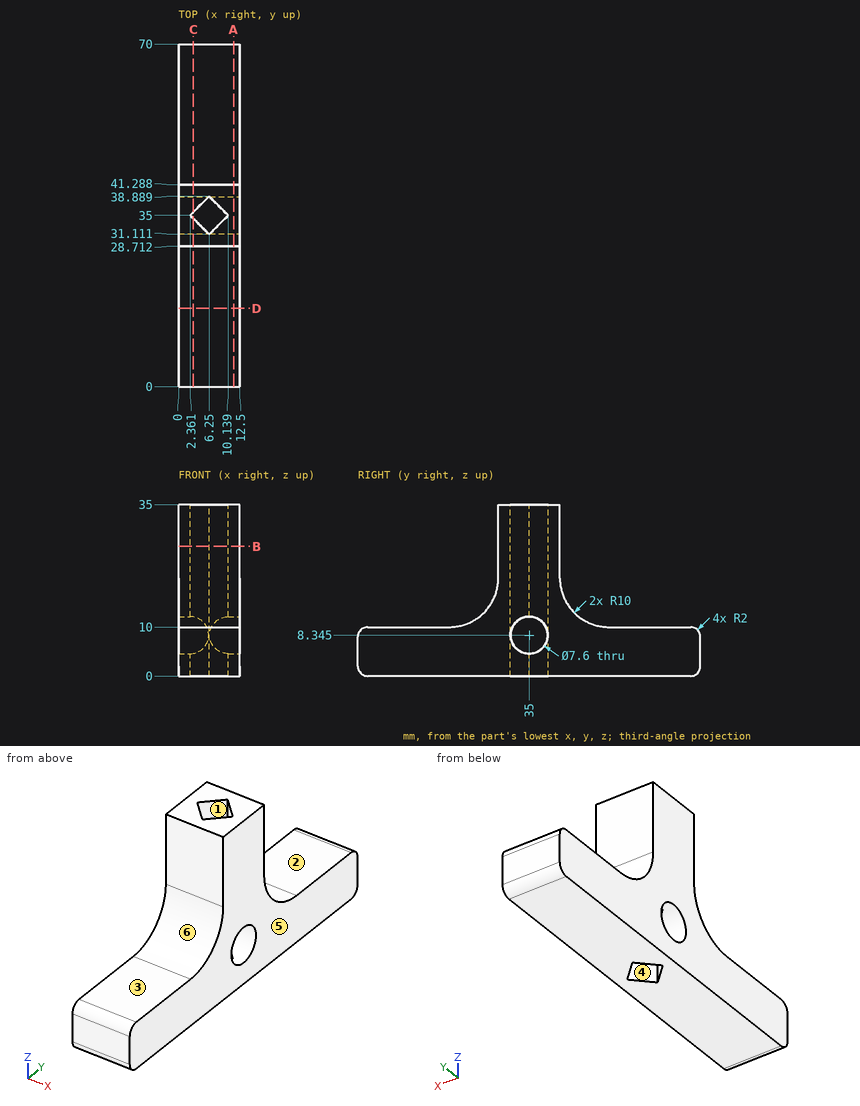
Could you check a few things on this drawing? It's one solid part, dimensions in mm from its lowest x, y, z. A direction names the side the tool comes from. Coordinates: 2 decimals unless noted, no trailing zeros. Loops run counter-clockwise (first coordinate to the right, second up) from the corner with the lowest first, then second, coordinate; pieces in that order, holes last. Notation, with made-up numbers: (67.5, -37) - (123.5, -37) arc R12 ccw to (123.5, -17) - close; hole circle Ø11 at (48, 76.5). An arc over 180 degrees is marked (long way). Answer as a JSON object with one key per item and string values. Group by question number.
Item 1: If we section it at C-C (x = 3): List the corners of the cut face in (y, z) for me (1 decimal).
Item 2: For pin 1 (4 mm diameter, centred on x = 8, y = 12, fed in from +Z); pin 2 (6 mm diameter, centred on x = 6, z = 24, fed in from -Y); pin 3 (1 mm diameter, centred on x = 10, z = 18.5, fed in from +Y); pin 4 (7 mm diameter, centred on y = 35, z = 8.34, fed in from +X), each with a flat end and sliding along its axis, tell me the tip position at first contact or that it passes through.
Item 3: On a 3-axis mill with a long thin cutter (end or side, diameter ignored), from which of +Z, -Z, +X, -X, +Y, -Y can I reach the whole of each face in a straight line? I mean the marked faces 1, 2 and 3. Say none if no direction works.
Item 4: If we section it at A-A (x = 11.25): List the corners of the cut face in (y, z) for me (1 decimal).
Item 5: If we section it at D-D (y = 16): List the corners of the cut face in (x, z) for me, plus the area to 3 significant figures.
Item 6: If I drill on L1, parallel to Z at x = 10.5, y = 35 (1 decimal); L2, parallel to X at y = 32, z = 20; L3, parallel to Z at x = 8, y = 59.5, over which ranges is the centre line in solid material (lowest first)? Write a range as from..to.
Item 7: If we mould it in two halves opening along X, with no side actions, what happens to the marked faces 4, 5 and 6? For each: released by +X, released by -X, zero draft, split by the parting line, or undercut.
Item 8: If we section it at B-B (z = 26.5): List the corners of the cut face in (x, y) for me.
Returned:
{
 "1": {"outline": "(0, 2) arc R2 ccw to (2, 0) - (34.4, 0) - (34.4, 4.6) arc R3.8 cw to (34.4, 12.1) - (34.4, 35) - (28.7, 35) - (28.7, 20) arc R10 cw to (18.7, 10) - (2, 10) arc R2 ccw to (0, 8) - close; (35.6, 0) - (68, 0) arc R2 ccw to (70, 2) - (70, 8) arc R2 ccw to (68, 10) - (51.3, 10) arc R10 cw to (41.3, 20) - (41.3, 35) - (35.6, 35) - (35.6, 12.1) arc R3.8 cw to (35.6, 4.6) - close"},
 "2": {"pin 1": "stops at z = 10", "pin 2": "stops at y = 28.71", "pin 3": "stops at y = 41.49", "pin 4": "passes through"},
 "3": {"face 1": "+Z, -Z", "face 2": "+Z, +X, -X, +Y", "face 3": "+Z, +X, -X, -Y"},
 "4": {"outline": "(0, 2) arc R2 ccw to (2, 0) - (68, 0) arc R2 ccw to (70, 2) - (70, 8) arc R2 ccw to (68, 10) - (51.3, 10) arc R10 cw to (41.3, 20) - (41.3, 35) - (28.7, 35) - (28.7, 20) arc R10 cw to (18.7, 10) - (2, 10) arc R2 ccw to (0, 8) - close; hole circle Ø7.6 at (35, 8.3)"},
 "5": {"outline": "(0, 0) - (12.5, 0) - (12.5, 10) - (0, 10) - close", "area": "125 mm²"},
 "6": {"L1": "z = 0..4.5, 12.1..35", "L2": "x = 0..5.36, 7.14..12.5", "L3": "z = 0..10"},
 "7": {"face 4": "undercut", "face 5": "released by +X", "face 6": "zero draft"},
 "8": {"outline": "(0, 28.71) - (12.5, 28.71) - (12.5, 41.29) - (0, 41.29) - close; hole (2.36, 35) - (6.25, 31.11) - (10.14, 35) - (6.25, 38.89) - close"}
}
